The drawing under review shows one solid part. Ordinate dimensions are in mm from its lowest x, y, z. Round coordinates to 2 decimals unless told otherwise and drop trailing zeros. Write each loop counter-clockwise with the first axis right and the second up, starting at its lowest first coordinate (ties: lowest second). Pieces come first, ordered by that corner, then holes. Notation, with made-up numbers: (42.25, 15.25) -> (64.25, 15.25) arc R26 cw to (64.25, 45.25) -> close; hole circle Ø3 at (80, 64.5). An arc over 180 degrees is marked (long way). Answer in a Markdown table with one row per item.
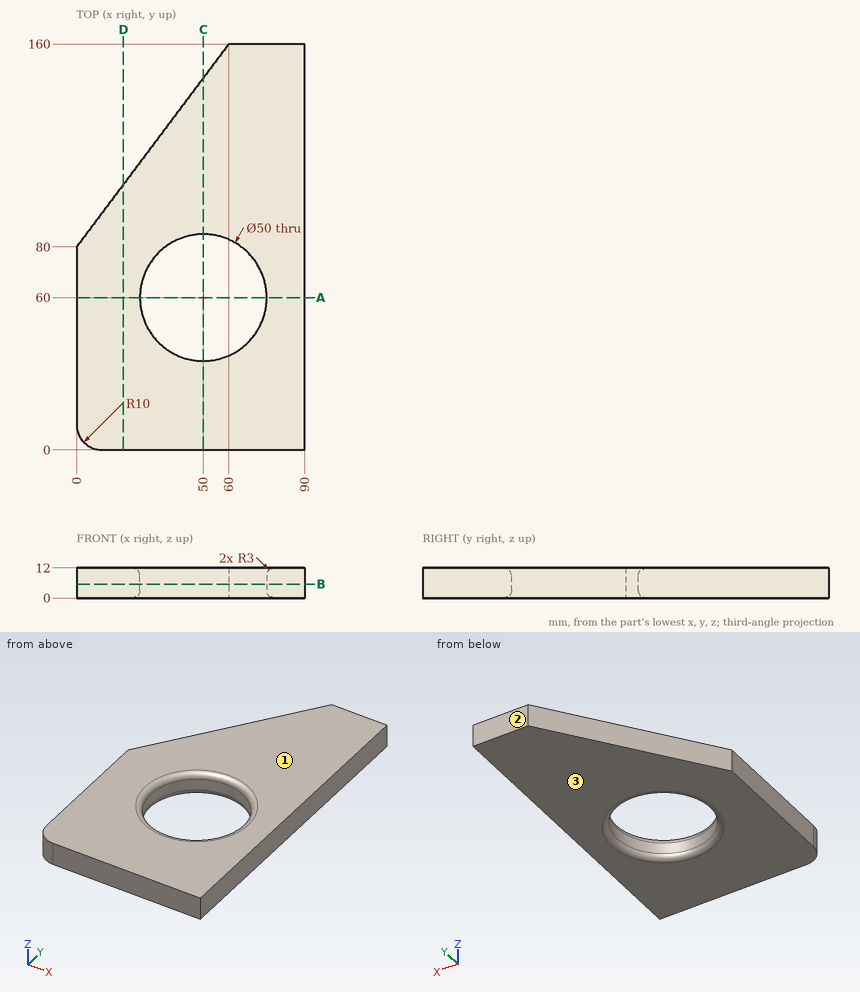
1) Consider section C-C on x = 50. State the section outline as (y, z) points.
Solved:
| item | result |
|---|---|
| outline | (0, 0) -> (32, 0) arc R3 ccw to (35, 3) -> (35, 9) arc R3 ccw to (32, 12) -> (0, 12) -> close; (85, 3) arc R3 ccw to (88, 0) -> (146.67, 0) -> (146.67, 12) -> (88, 12) arc R3 ccw to (85, 9) -> close |
2) Consider section D-D on x = 18.5. State the section outline as (y, z) points, then the cut area to 3 significant figures.
Solved:
| item | result |
|---|---|
| outline | (0, 0) -> (104.67, 0) -> (104.67, 12) -> (0, 12) -> close |
| area | 1,260 mm² |
3) Mouldability with a two-part tool opening along Z and no side actions: class the marked faces 1, 2 and 3 as pulls with the +Z half, pulls with the -Z half, needs draft (parallel to the pull), parting line crosses it, or undercut.
Solved:
| item | result |
|---|---|
| face 1 | pulls with the +Z half |
| face 2 | needs draft |
| face 3 | pulls with the -Z half |
4) Consider section A-A on y = 60. State the section outline as (x, z) points.
Solved:
| item | result |
|---|---|
| outline | (0, 0) -> (22, 0) arc R3 ccw to (25, 3) -> (25, 9) arc R3 ccw to (22, 12) -> (0, 12) -> close; (75, 3) arc R3 ccw to (78, 0) -> (90, 0) -> (90, 12) -> (78, 12) arc R3 ccw to (75, 9) -> close |
5) Consider section B-B on z = 5.5. State the section outline as (x, y) points.
Solved:
| item | result |
|---|---|
| outline | (0, 10) arc R10 ccw to (10, 0) -> (90, 0) -> (90, 160) -> (60, 160) -> (0, 80) -> close; hole circle Ø50 at (50, 60) |
6) For line 1 (X direction, y = 51, z = 5.25); line 2 (Y direction, x = 50, z = 7.7); line 3 (Y direction, x = 30.5, z = 11.25), list the stretches that pass through material, from the lowest coordinate up. Write a range as [from, to].
Solved:
| item | result |
|---|---|
| line 1 | [0, 26.68], [73.32, 90] |
| line 2 | [0, 35], [85, 146.67] |
| line 3 | [0, 42.78], [77.22, 120.67] |
7) Clearance check with a flat-ended pin moving along its axis: pin 1 Ø1 at (x, y) = (39, 83) entering from +Z. State where the tip first meets the part, or that it passes through.
Solved:
| item | result |
|---|---|
| pin 1 | z = 11.23 |
